```python
from build123d import *

# Parameters (mm, degrees)
SKETCH1_R           = 11
SKETCH1_R_2         = 4.25
BOSS_EXTRUDE1_DEPTH = 4
SKETCH2_R           = 1.4
CUT_EXTRUDE1_DEPTH  = 17.062378404
SKETCH3_R           = 7.5
BOSS_EXTRUDE2_DEPTH = 2
SKETCH4_R           = 2.811136831
CUT_EXTRUDE2_DEPTH  = 2
SKETCH5_R           = 4.5
BOSS_EXTRUDE3_DEPTH = 7
CUT_EXTRUDE3_START  = -6
SKETCH6_R           = 4.5
SKETCH6_R_2         = 4
CUT_EXTRUDE3_DEPTH  = 6
BOSS_EXTRUDE4_DEPTH = 4
SKETCH13_W          = 22
SKETCH13_H          = 3.5
BOSS_EXTRUDE5_DEPTH = 46.25
SKETCH14_W          = 22
SKETCH14_H          = 5.5
BOSS_EXTRUDE6_DEPTH = 45
CUT_EXTRUDE6_START  = -30
SKETCH16_R          = 4.25
SKETCH16_R_2        = 1.4
CUT_EXTRUDE6_DEPTH  = 30
SKETCH17_W          = 9.75
SKETCH17_H          = 5.5
BOSS_EXTRUDE7_DEPTH = 20
FILLET3_R           = 2
SKETCH19_R          = 2.5
CUT_EXTRUDE8_DEPTH  = 1.5
SKETCH21_W          = 3.5
SKETCH21_H          = 40.2
BOSS_EXTRUDE8_DEPTH = 61.1
SKETCH22_R          = 1.4
SKETCH22_W          = 29.3
SKETCH22_H          = 55.6
CUT_EXTRUDE10_DEPTH = 61.1
FILLET4_R           = 5
FILLET5_R           = 3


with BuildPart() as part:
    # Sketch1 → Boss-Extrude1 (new body)
    with BuildSketch(Plane(origin=(0, 0, 0), x_dir=(1, 0, 0), z_dir=(0, 1, 0))):
        with Locations(Location((0, 0, 0), (0, 0, 270))):
            Circle(SKETCH1_R)
        with Locations(Location((0, 0, 0), (0, 0, 270))):
            Circle(SKETCH1_R_2, mode=Mode.SUBTRACT)
    extrude(amount=BOSS_EXTRUDE1_DEPTH)

    # Sketch2 → Cut-Extrude1 (cut, through all)
    with BuildSketch(Plane(origin=(0, 4, 0), x_dir=(1, 0, 0), z_dir=(0, 1, 0))):
        with Locations(Location((0, 8, 0), (0, 0, 270))):
            Circle(SKETCH2_R)
        with Locations(Location((8, 0, 0), (0, 0, 270))):
            Circle(SKETCH2_R)
        with Locations(Location((0, -8, 0), (0, 0, 270))):
            Circle(SKETCH2_R)
        with Locations(Location((-8, 0, 0), (0, 0, 270))):
            Circle(SKETCH2_R)
    extrude(amount=-CUT_EXTRUDE1_DEPTH, mode=Mode.SUBTRACT)

    # Sketch3 → Boss-Extrude2 (add)
    with BuildSketch(Plane(origin=(0, 4, 0), x_dir=(1, 0, 0), z_dir=(0, 1, 0))):
        with Locations(Location((0, 0, 0), (0, 0, 80.315835906))):
            Circle(SKETCH3_R)
    extrude(amount=BOSS_EXTRUDE2_DEPTH)

    # Sketch4 → Cut-Extrude2 (cut)
    with BuildSketch(Plane(origin=(0, 6, 0), x_dir=(1, 0, 0), z_dir=(0, 1, 0))):
        with Locations((8, 0)):
            Circle(SKETCH4_R)
        with Locations((0, -8)):
            Circle(SKETCH4_R)
        with Locations((-8, 0)):
            Circle(SKETCH4_R)
        with Locations((0, 8)):
            Circle(SKETCH4_R)
    extrude(amount=-CUT_EXTRUDE2_DEPTH, mode=Mode.SUBTRACT)

    # Sketch5 → Boss-Extrude3 (add)
    with BuildSketch(Plane(origin=(0, 6, 0), x_dir=(1, 0, 0), z_dir=(0, 1, 0))):
        with Locations(Location((0, 0, 0), (0, 0, 270))):
            Circle(SKETCH5_R)
    extrude(amount=BOSS_EXTRUDE3_DEPTH)

    # Sketch6 → Cut-Extrude3 (cut)
    with BuildSketch(Plane(origin=(0, 13, 0), x_dir=(1, 0, 0), z_dir=(0, 1, 0)).offset(CUT_EXTRUDE3_START)):
        with Locations(Location((0, 0, 0), (0, 0, 270))):
            Circle(SKETCH6_R)
        with Locations(Location((0, 0, 0), (0, 0, 270))):
            Circle(SKETCH6_R_2, mode=Mode.SUBTRACT)
    extrude(amount=CUT_EXTRUDE3_DEPTH, mode=Mode.SUBTRACT)

    # Sketch8 → Boss-Extrude4 (add)
    with BuildSketch(Plane.XZ):
        with BuildLine():
            Line((11, 30), (-11, 30))
            Line((-11, 30), (-11, 0))
            ThreePointArc((-11, 0), (0, 11), (11, 0))
            Line((11, 0), (11, 30))
        make_face()
    extrude(amount=-BOSS_EXTRUDE4_DEPTH)

    # Sketch13 → Boss-Extrude5 (add)
    with BuildSketch(Plane(origin=(0, 4, 0), x_dir=(1, 0, 0), z_dir=(0, 1, 0))):
        with Locations((0, -31.75)):
            Rectangle(SKETCH13_W, SKETCH13_H)
    extrude(amount=-BOSS_EXTRUDE5_DEPTH)

    # Sketch14 → Boss-Extrude6 (add)
    with BuildSketch(Plane.XY.offset(33.5)):
        with Locations((0, -45)):
            Rectangle(SKETCH14_W, SKETCH14_H)
    extrude(amount=-BOSS_EXTRUDE6_DEPTH)

    # Sketch16 → Cut-Extrude6 (cut)
    with BuildSketch(Plane.XZ.offset(47.75).offset(CUT_EXTRUDE6_START)):
        with Locations(Location((0, 0, 0), (0, 0, 90))):
            Circle(SKETCH16_R)
        with Locations(Location((-8, 0, 0), (0, 0, 90))):
            Circle(SKETCH16_R_2)
        with Locations(Location((0, -8, 0), (0, 0, 90))):
            Circle(SKETCH16_R_2)
        with Locations(Location((8, 0, 0), (0, 0, 90))):
            Circle(SKETCH16_R_2)
        with Locations(Location((0, 8, 0), (0, 0, 90))):
            Circle(SKETCH16_R_2)
    extrude(amount=CUT_EXTRUDE6_DEPTH, mode=Mode.SUBTRACT)

    # Sketch17 → Boss-Extrude7 (add)
    with BuildSketch(Plane(origin=(0, 0, -11.5), x_dir=(-1, 0, 0), z_dir=(0, 0, -1))):
        with Locations((-15.875, -45)):
            Rectangle(SKETCH17_W, SKETCH17_H)
        with Locations((15.875, -45)):
            Rectangle(SKETCH17_W, SKETCH17_H)
    extrude(amount=-BOSS_EXTRUDE7_DEPTH)

    # Fillet3
    fillet3_edges = [part.edges().sort_by_distance(p)[0] for p in [
        (0, 0, 30),
        (0, -42.25, 30),
        (0, 4, 33.5),
        (0, -47.75, 33.5),
    ]]
    fillet(fillet3_edges, radius=FILLET3_R)

    # Sketch19 → Cut-Extrude8 (cut)
    with BuildSketch(Plane.XZ.offset(47.75)):
        with Locations((-8, 0)):
            Circle(SKETCH19_R)
        with Locations((0, 8)):
            Circle(SKETCH19_R)
        with Locations((8, 0)):
            Circle(SKETCH19_R)
        with Locations((0, -8)):
            Circle(SKETCH19_R)
    extrude(amount=-CUT_EXTRUDE8_DEPTH, mode=Mode.SUBTRACT)

    # Sketch21 → Boss-Extrude8 (add)
    with BuildSketch(Plane.XZ.offset(47.75)):
        with Locations((-19, 0)):
            Rectangle(SKETCH21_W, SKETCH21_H)
        with Locations((19, 0)):
            Rectangle(SKETCH21_W, SKETCH21_H)
    extrude(amount=BOSS_EXTRUDE8_DEPTH)

    # Sketch22 → Cut-Extrude10 (cut)
    with BuildSketch(Plane(origin=(20.75, 0, 0), x_dir=(0, 0, -1), z_dir=(1, 0, 0))):
        with Locations((-11, -50.5)):
            Circle(SKETCH22_R)
        with Locations((11, -50.5)):
            Circle(SKETCH22_R)
        with Locations((-17.375, -99.85)):
            Circle(SKETCH22_R)
        with Locations((-17.375, -77.85)):
            Circle(SKETCH22_R)
        with Locations((-17.375, -55.85)):
            Circle(SKETCH22_R)
        with Locations((17.375, -99.85)):
            Circle(SKETCH22_R)
        with Locations((17.375, -77.85)):
            Circle(SKETCH22_R)
        with Locations((17.375, -55.85)):
            Circle(SKETCH22_R)
        with Locations((0, -81.05)):
            Rectangle(SKETCH22_W, SKETCH22_H)
    extrude(amount=-CUT_EXTRUDE10_DEPTH, mode=Mode.SUBTRACT)

    # Fillet4
    fillet4_edges = [part.edges().sort_by_distance(p)[0] for p in [
        (11, -45, 8.5),
        (-11, -45, 8.5),
    ]]
    fillet(fillet4_edges, radius=FILLET4_R)

    # Fillet5
    fillet5_edges = [part.edges().sort_by_distance(p)[0] for p in [
        (-19, -47.75, -11.5),
        (19, -47.75, 8.5),
        (-19, -47.75, 8.5),
        (19, -47.75, -11.5),
    ]]
    fillet(fillet5_edges, radius=FILLET5_R)


solid = part.part
```
Work out the finished part from the listing and answer in its coordinate system (mm). A direction names the side the tool comes from. Round coordinates to 2 decimals unless told otherwise and drop trailing zeros. Loops run counter-clockwise (first coordinate to the right, second up) from the corner with the lowest first, then second, coordinate; pieces in that order, holes last. Notation, with made-up numbers: (8, -14.75) -> (26, -14.75) arc R19 ccw to (26, 16.25) -> close; hole circle Ø2 at (-13, 51.25). An arc over 180 degrees is marked (long way). Write each question's results on one line, items separated by ' | '. Start each with the question number.
1. Find the intervals of material crossed by probe 1 along X at (y, z) = (0.8, 0); probe 2 along Y at (x, z) = (-9, -2); probe 3 along Y at (x, z) = (-4, 18), in increasing order. Write a range as from..to.
2. Section A-A (y = -50.5) is taken. Determine the outline of the cut face in (x, z).
3. Given pin 1 Ø8 at (x, y) = (-7.5, -34) entering from -Z; pin 2 Ø1 at (x, z) = (-4, 25.5) entering from +Y; pin 3 Ø6 at (x, z) = (-8, 0) entering from -Y, each flat-ended and moving along its own axis, determine where each tip first touches the part or whether it passes through.
4. Section B-B (x = 0) is taken. State how many separate pieces and enclosed holes the cut face has, plus the area to 3 significant figures.
5. Section C-C (y = -36) is taken. Determine the outline of the cut face in (x, z), plus the area to 3 significant figures.
6. For a pull along X with two mould halves and no side action, classify faces 4 (the face through (19, -78, -20.1)), 5 (the face through (1.1, -46.25, 6.9)), 6 (the face through (-20.75, -73, -15)), 7 (the face through (-3.905, 9.958, -0.867)) as +X half, -X half, draft (parallel to the pull), parting line (faces both ways), or undercut.
7. A tool of negligible diameter and unlimited length cuts with its end or side. For faces 1 (the face through (1.1, -46.25, -9.1)), 2 (the face through (19, -47.75, -17)), 3 (the face through (0, -47.75, 5)), from which of +Z, -Z, +X, -X, +Y, -Y can it reach the whole face along a straight path? Write none if from no direction.
8. Section D-D (x = 13.5) is taken. Determine the outline of the cut face in (y, z).
Evaluation:
1) probe 1: x = -11..-9.4, -6.6..-4.25, 4.25..6.6, 9.4..11 | probe 2: y = -46.25..-42.25, 0..4 | probe 3: y = -47.75..-42.25, 0..4
2) outline: (-20.75, -20.1) -> (-17.25, -20.1) -> (-17.25, -12.4) -> (-20.75, -12.4) -> close; (-20.75, -9.6) -> (-17.25, -9.6) -> (-17.25, 9.6) -> (-20.75, 9.6) -> close; (-20.75, 12.4) -> (-17.25, 12.4) -> (-17.25, 20.1) -> (-20.75, 20.1) -> close; (17.25, -20.1) -> (20.75, -20.1) -> (20.75, -12.4) -> (17.25, -12.4) -> close; (17.25, -9.6) -> (20.75, -9.6) -> (20.75, 9.6) -> (17.25, 9.6) -> close; (17.25, 12.4) -> (20.75, 12.4) -> (20.75, 20.1) -> (17.25, 20.1) -> close
3) pin 1: stops at z = 30 | pin 2: stops at y = 4 | pin 3: stops at y = -47.75
4) separate pieces: 6 | enclosed holes: 0 | area: 511 mm2
5) outline: (-11, 30) -> (11, 30) -> (11, 33.5) -> (-11, 33.5) -> close | area: 77.0 mm2
6) face 4: draft | face 5: undercut | face 6: -X half | face 7: parting line
7) face 1: -Y | face 2: -Z, +X, -X, +Y | face 3: +Z, -Z, -Y
8) outline: (-47.75, -11.5) -> (-42.25, -11.5) -> (-42.25, 9.17) -> (-47.75, 9.17) -> close
